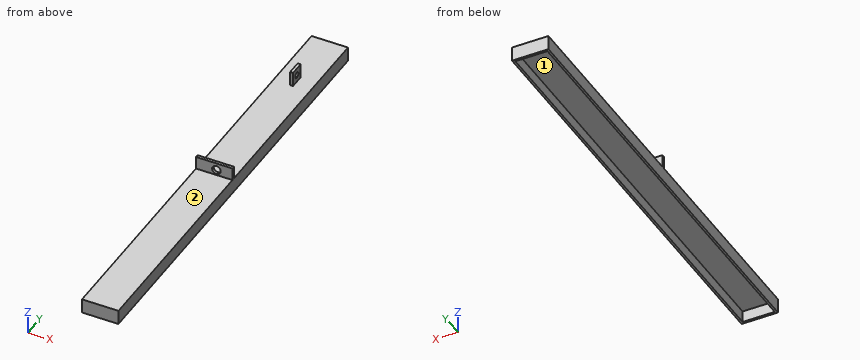
from build123d import *

# Parameters (mm, degrees)
SKETCH1_W           = 25
SKETCH1_H           = 300
SKETCH1_W_2         = 22
SKETCH1_H_2         = 297
BOSS_EXTRUDE1_DEPTH = 10
SKETCH3_W           = 22
SKETCH3_H           = 297
BOSS_EXTRUDE2_DEPTH = 1.5
BOSS_EXTRUDE3_DEPTH = 25
SKETCH7_R           = 2.959313076
CUT_EXTRUDE1_DEPTH  = 2
SKETCH9_W           = 2
SKETCH9_H           = 10
BOSS_EXTRUDE4_DEPTH = 10
SKETCH10_R          = 2
CUT_EXTRUDE2_DEPTH  = 15
SKETCH11_W          = 22
SKETCH11_H          = 297
CUT_EXTRUDE7_DEPTH  = 8


with BuildPart() as part:
    # Sketch1 → Boss-Extrude1 (new body)
    with BuildSketch(Plane.XY):
        with Locations((-21.911764706, -122.5)):
            Rectangle(SKETCH1_W, SKETCH1_H)
        with Locations((-21.911764706, -122.5)):
            Rectangle(SKETCH1_W_2, SKETCH1_H_2, mode=Mode.SUBTRACT)
    extrude(amount=BOSS_EXTRUDE1_DEPTH)

    # Sketch3 → Boss-Extrude2 (add)
    with BuildSketch(Plane.XY.offset(10)):
        with Locations((-21.911764706, -122.5)):
            Rectangle(SKETCH3_W, SKETCH3_H)
    extrude(amount=-BOSS_EXTRUDE2_DEPTH)

    # Sketch6 → Boss-Extrude3 (add)
    with BuildSketch(Plane.ZY.offset(34.411764706)):
        Polygon((10, -121.5), (18.820577113, -121.5), (18.820577113, -123.5), (10, -123.5), (10, -272.5), (0, -272.5), (0, 27.5), (10, 27.5), align=None)
    extrude(amount=-BOSS_EXTRUDE3_DEPTH)

    # Sketch7 → Cut-Extrude1 (cut)
    with BuildSketch(Plane.XZ.offset(123.5)):
        with Locations(Location((-20.411764706, 13.820577113, 0), (0, 0, 270))):
            Circle(SKETCH7_R)
    extrude(amount=-CUT_EXTRUDE1_DEPTH, mode=Mode.SUBTRACT)

    # Sketch9 → Boss-Extrude4 (add)
    with BuildSketch(Plane.XY.offset(10)):
        with Locations((-21.911764706, -17.5)):
            Rectangle(SKETCH9_W, SKETCH9_H)
    extrude(amount=BOSS_EXTRUDE4_DEPTH)

    # Sketch10 → Cut-Extrude2 (cut)
    with BuildSketch(Plane.ZY.offset(34.411764706)):
        with Locations((15, -17.5)):
            Circle(SKETCH10_R)
    extrude(amount=-CUT_EXTRUDE2_DEPTH, mode=Mode.SUBTRACT)

    # Sketch11 → Cut-Extrude7 (cut)
    with BuildSketch(Plane(origin=(0, 0, 0), x_dir=(-1, 0, 0), z_dir=(0, 0, -1))):
        with Locations((21.911764706, -122.5)):
            Rectangle(SKETCH11_W, SKETCH11_H)
    extrude(amount=-CUT_EXTRUDE7_DEPTH, mode=Mode.SUBTRACT)


solid = part.part
Design review of the part built by this model. Coordinates are the model's own, in mm. Face numbers are marked on the shaded views. Round coordinates to 2 decimals unless told otherwise and drop trailing zeros. Write each loop counter-clockwise with the first axis right and the second up, starting at its lowest first coordinate (ties: lowest second). Pieces come first, ordered by that corner, then holes. Notation, with made-up numbers: (40.25, 34.5) - (59.25, 34.5) arc R29 ccw to (59.25, 58.5) - close; hole circle Ø7 at (85.5, 13.5). An arc over 180 degrees is marked (long way). Use a Markdown table: item, result. Add a question column.
1. Wall thickness on probe 1 along X at (y, z) = (-185, 3); probe 2 along Y at (x, z) = (-22.15, 15); probe 3 along Z at (x, y) = (-16.5, -18): over which ranges is each line inside the solid? List them lowest first.
2. We need section A-A (y = -67). State the section outline as (x, z) points, then the cut area to 3 significant figures.
3. Clearance check with flat-ended pins moving along their axes: pin 1 (2 mm diameter, centred on x = -22.5, z = 15.5, fed in from +Y); pin 2 (3 mm diameter, centred on y = -22.5, z = 17, fed in from +X); pin 3 (5 mm diameter, centred on y = -15.5, z = 15.5, fed in from -X). State where each tip first meets the part, or that it passes through.
4. Mouldability with a two-part tool opening along Y and no side actions: class the marked faces 1 and 2 as +Y half, -Y half, draft (parallel to the pull), parting line (faces both ways), or undercut.
Output:
| question | item | result |
|---|---|---|
| 1 | probe 1 | x = -34.41 to -32.91, -10.91 to -9.41 |
| 1 | probe 2 | y = -22.5 to -19.5, -15.5 to -12.5 |
| 1 | probe 3 | z = 8 to 10 |
| 2 | outline | (-34.41, 0) - (-32.91, 0) - (-32.91, 8) - (-10.91, 8) - (-10.91, 0) - (-9.41, 0) - (-9.41, 10) - (-34.41, 10) - close |
| 2 | area | 74.0 mm2 |
| 3 | pin 1 | stops at y = -12.5 |
| 3 | pin 2 | stops at x = -20.91 |
| 3 | pin 3 | stops at x = -22.91 |
| 4 | face 1 | undercut |
| 4 | face 2 | draft |
